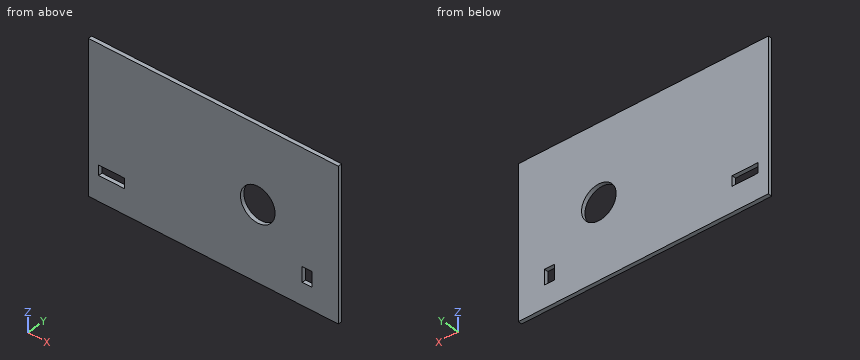
from build123d import *

# Parameters (mm, degrees)
SKETCH2_W           = 253
SKETCH2_H           = 150
BOSS_EXTRUDE1_DEPTH = 4
SKETCH3_R           = 17.5
SKETCH3_W           = 26
SKETCH3_H           = 10
SKETCH3_W_2         = 10
SKETCH3_H_2         = 15
CUT_EXTRUDE1_DEPTH  = 148.116450474


with BuildPart() as part:
    # Sketch2 → Boss-Extrude1 (new body)
    with BuildSketch(Plane(origin=(0, 0, 0), x_dir=(1, 0, 0), z_dir=(0, 1, 0))):
        Rectangle(SKETCH2_W, SKETCH2_H)
    extrude(amount=BOSS_EXTRUDE1_DEPTH)

    # Sketch3 → Cut-Extrude1 (cut, through all)
    with BuildSketch(Plane(origin=(0, 4, 0), x_dir=(1, 0, 0), z_dir=(0, 1, 0))):
        with Locations(Location((45, 0.713202338, 0), (0, 0, 270))):
            Circle(SKETCH3_R)
        with Locations((-103, 45.288057663)):
            Rectangle(SKETCH3_W, SKETCH3_H)
        with Locations((95, 45.445405543)):
            Rectangle(SKETCH3_W_2, SKETCH3_H_2)
    extrude(amount=-CUT_EXTRUDE1_DEPTH, mode=Mode.SUBTRACT)


solid = part.part
Design review of the part built by this model. Coordinates are the model's own, in mm. Give positions to 0.01 mm unless a question says otherwise; leave off trailing zeros. Write each loop counter-clockwise with the first axis right and the second up, starting at its lowest first coordinate (ties: lowest second). Pieces come first, ordered by that corner, then holes. Notation, with made-up numbers: M -9.5,-38.75 L 41.5,-38.75 A33 cw 41.5,-4.75 Z; hole C 10,-39.75 d5. An arc over 180 degrees is marked long. Return JSON: item names as keys, results as strings. Group by question number.
Item 1: Take a section at A-A (x = 45). Give the boundary of the cut face in (y, z).
Item 2: Wall thickness on line 1 along X through (y, z) = (0.85, -45); line 2 along X through (y, z) = (2.65, -38); line 3 along X through (y, z) = (3.55, 6.5): over which ranges is each line inside the solid? List them lowest first.
Item 3: Clearance check with a flat-ended pin moving along its axis: pin 1 Ø1 at (x, z) = (44, -21) entering from -Y. State where the tip first meets the part, or that it passes through.
Item 4: Take a section at C-C (y = 1.7). Give the boundary of the cut face in (x, z).
Item 5: Take a section at B-B (z = -4). Give the boundary of the cut face in (x, y), plus the area to 3 significant figures.
Return value:
{
 "1": {"outline": "M 0,-75 L 4,-75 L 4,-18.21 L 0,-18.21 Z; M 0,16.79 L 4,16.79 L 4,75 L 0,75 Z"},
 "2": {"line 1": "x = -126.5 to -116, -90 to 90, 100 to 126.5", "line 2": "x = -126.5 to 90, 100 to 126.5", "line 3": "x = -126.5 to 29.06, 60.94 to 126.5"},
 "3": {"pin 1": "stops at y = 0"},
 "4": {"outline": "M -126.5,-75 L 126.5,-75 L 126.5,75 L -126.5,75 Z; hole M -116,-50.29 L -90,-50.29 L -90,-40.29 L -116,-40.29 Z; hole C 45,-0.71 d35; hole M 90,-52.95 L 100,-52.95 L 100,-37.95 L 90,-37.95 Z"},
 "5": {"outline": "M -126.5,0 L 27.81,0 L 27.81,4 L -126.5,4 Z; M 62.19,0 L 126.5,0 L 126.5,4 L 62.19,4 Z", "area": "874 mm2"}
}
